Input: part model. Units: mm. Frame: model coordinates. Face numbers are marked on the shaded views. Give positions to 0.01 mm unless a question says otherwise; leave off trailing zeros. Loops run counter-clockwise (first coordinate to the right, second up) from the corner with the lowest first, then second, coordinate; pieces in that order, holes last. Notation, with made-up numbers: (-28.75, 17.25) - (-16.75, 17.25) arc R22 ccw to (-16.75, 30.25) - close; hole circle Ø8 at (-4, 71.5). An arc over 180 degrees is marked (long way). One line per question, with ' | ' between items. Start each with the question number.
from build123d import *

# Parameters (mm, degrees)
F1_DEPTH  = 2
F2_R      = 3
F3_DEPTH  = 2
F4_W      = 2
F4_H      = 3
F5_DEPTH  = 5
F6_R      = 2.5
F7_R      = 1.49999
F8_R      = 0.5
F10_DEPTH = 5
F12_DEPTH = 2
F13_R     = 9.9401429079
F13_R_2   = 5
F14_DEPTH = 1.7623205361
F16_DEPTH = 1.7623205361
F17_R     = 2


# Not quite as in the source:
# - a fillet or chamfer is up to 0.001 mm smaller than in the source, because OpenCascade refuses the exact size


with BuildPart() as f1:
    # F0 (on Top) → F1 (new body)
    with BuildSketch(Plane.XY):
        Polygon((-19.7472184807, 28), (-19.7472184807, 0), (26.2527815193, 0), (26.2527815193, 6), (-14.7472184807, 28), align=None)
    extrude(amount=F1_DEPTH)

    # F2 (on face) → F3 (cut, through all)
    with BuildSketch(Plane.XY.offset(2)):
        with Locations((-13.5472184807, 7)):
            Circle(F2_R)
        with Locations((4.4527815193, 7)):
            Circle(F2_R)
        with BuildLine():
            Line((-9.5472184807, 7), (-9.5472184807, 0))
            Line((-9.5472184807, 0), (0.4527815193, 0))
            Line((0.4527815193, 0), (0.4527815193, 7))
            ThreePointArc((0.4527815193, 7), (-4.5472184807, 12), (-9.5472184807, 7))
        make_face()
    extrude(amount=-F3_DEPTH, mode=Mode.SUBTRACT)

    # F4 (on face) → F5 (join)
    with BuildSketch(Plane(origin=(8.3687511572, 15.5963089748, 0), x_dir=(-0.8811602681, 0.4728177048, 0), z_dir=(0.4728177048, 0.8811602681, 0))):
        Polygon((3.5210567079, 2), (5.5210567079, 2), (5.5210567079, 10), (-6.4789432921, 10), (-6.4789432921, 5.0490344875), (-4.4789432921, 5.0490344875), (-4.4789432921, 8), (3.5210567079, 8), align=None)
        with Locations((-0.4789432921, 3.5)):
            Rectangle(F4_W, F4_H)
    extrude(amount=-F5_DEPTH)

    # F6
    f6_edges = [f1.edges().sort_by_distance(p)[0] for p in [
        (12.895694, 10.330049, 10),
        (2.321771, 16.003862, 10),
    ]]
    fillet(f6_edges, radius=F6_R)

    # F7 (radius 1.5 in the source; OpenCascade refuses exactly that, so slightly less here)
    f7_edges = [f1.edges().sort_by_distance(p)[0] for p in [
        (6.727572, 13.639773, 2),
        (4.084092, 15.058226, 2),
        (11.133374, 11.275685, 8),
        (4.084092, 15.058226, 8),
    ]]
    fillet(f7_edges, radius=F7_R)

    # F8
    f8_edges = [f1.edges().sort_by_distance(p)[0] for p in [
        (12.895694, 10.330049, 5.049034),
        (11.133374, 11.275685, 5.049034),
        (8.489893, 12.694138, 5),
        (6.727572, 13.639773, 5),
    ]]
    fillet(f8_edges, radius=F8_R)

    # F9 (on face) → F10 (join)
    with BuildSketch(Plane(origin=(0, 0, 0), x_dir=(1, 0, 0), z_dir=(0, 0, -1))):
        Polygon((-19.7472184807, -26), (-19.7472184807, -28), (-14.7472184807, -28), (26.2527815193, -6), (26.2527815193, -4), (-14.7472184807, -26), align=None)
    extrude(amount=F10_DEPTH)

    # F11 (on face) → F12 (join)
    with BuildSketch(Plane(origin=(0, 0, -5), x_dir=(1, 0, 0), z_dir=(0, 0, -1))):
        Polygon((-15.9292627427, -23.7970993298), (-14.7472184807, -26), (1.1136663445, -17.4892813133), (-4.4741792579, -17.6504691673), align=None)
        Polygon((8.6295761581, -13.4563540963), (23.1687205811, -5.6548619669), (21.105516051, -3.9247790015), (8.7692722981, -10.5442268689), align=None)
    extrude(amount=-F12_DEPTH)

    # F13 (on face) → F14 (join, through all)
    with BuildSketch(Plane(origin=(8.3687511572, 15.5963089748, 0), x_dir=(-0.8811602681, 0.4728177048, 0), z_dir=(0.4728177048, 0.8811602681, 0))):
        with Locations((-29.5995731847, -1.5)):
            Circle(F13_R)
        with Locations((-29.5995731847, -1.5)):
            Circle(F13_R_2, mode=Mode.SUBTRACT)
    extrude(amount=-F14_DEPTH)

    # F15 (on face) → F16 (cut, through all)
    with BuildSketch(Plane(origin=(8.3687511572, 15.5963089748, 0), x_dir=(-0.8811602681, 0.4728177048, 0), z_dir=(0.4728177048, 0.8811602681, 0))):
        with BuildLine():
            ThreePointArc((-34.5031041583, -2.4774374616), (-34.5995731847, -1.5), (-34.5031041583, -0.5225625384))
            Line((-34.5031041583, -0.5225625384), (-39.4258868897, 0))
            ThreePointArc((-39.4258868897, 0), (-39.5397160926, -1.5), (-39.4258868897, -3))
            Line((-39.4258868897, -3), (-34.5031041583, -2.4774374616))
        make_face()
    extrude(amount=-F16_DEPTH, mode=Mode.SUBTRACT)

    # F17
    f17_edges = [f1.edges().sort_by_distance(p)[0] for p in [
        (42.692648, -3.821392, -3),
        (42.692648, -3.821392, 0),
        (38.354887, -1.493813, -0.522563),
        (38.354887, -1.493813, -2.477437),
    ]]
    fillet(f17_edges, radius=F17_R)


solid = f1.part
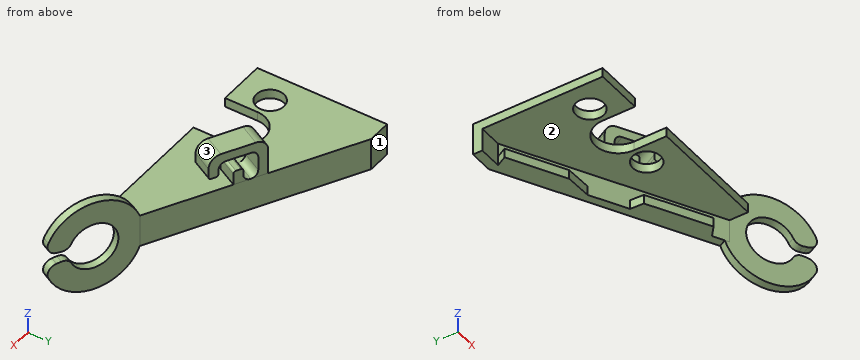
Q1. Section B-B, the plane z = -1.5. Output: boundary loops of the cut face in (x, y), plus the area to 3 significant figures.
Q2. First-contact query: pin 1 (1.6 mm diameter, centred on y = 3.5, z = 1.5, fed in from +X); pin 2 (4.5 mm diameter, centred on x = -3, y = 20, fed in from +Z); pin 3 (2 mm diameter, centred on x = 12, z = 1, fed in from -Y); pin 4 (5.5 mm diameter, centred on x = 4.45, y = 7, fed in from +Z). Flat tips, straight axial feed; report the tip coordinate or a pass-through.
Q3. Draft query along Y for the marked faces 1, 2 and 3. Return one class per face: +Y half, -Y half, draft (parallel to the pull), parting line (faces both ways), or undercut.
Q4. Section A-A, the plane y = 22. Output: boundary loops of the cut face in (x, z), plus the area to 3 significant figures.
Q5. Line query: L1, parallel to Z at x = 18, y = 7.5; L2, parallel to Z at x = -4, y = 21.5; L3, parallel to Z at x = 2, y = 13. Output: solid intervals per line, ascending. Write a range as from..to.
Solved:
1) outline: (-19.75, 26) - (-14.75, 26) - (29.21, 2.41) - (30.04, 3.97) - (-14.75, 28) - (-19.75, 28) - close | area: 98.8 mm²
2) pin 1: stops at x = 31.52 | pin 2: stops at z = 2 | pin 3: stops at y = 0 | pin 4: passes through
3) face 1: +Y half | face 2: draft | face 3: -Y half
4) outline: (-19.75, 0) - (-7.29, 0) - (-7.29, -3) - (-12.58, -3) - (-12.58, -5) - (-3.57, -5) - (-3.57, 2) - (-19.75, 2) - close | area: 61.6 mm²
5) L1: z = -5..-3, 0..2 | L2: z = -5..2 | L3: z = 0..2
